```python
from build123d import *

# Parameters (mm, degrees)
EXTRUDE1_DEPTH  = 3
LPATTERN1_COUNT = 2
LPATTERN1_PITCH = 13.06


with BuildPart() as part:
    # Sketch1 → Extrude1 (new body)
    with BuildSketch(Plane(origin=(0, 0, 0), x_dir=(1, 0, 0), z_dir=(0, 1, 0))):
        Polygon((11.547005384, 0), (-5.773502692, 10), (-5.773502692, -10), align=None)
    extrude(amount=EXTRUDE1_DEPTH)

    # Sketch6 → #2-56 Tapped Hole1 (revolve, cut)
    with BuildSketch(Plane(origin=(-3.77, 3, -6.53), x_dir=(0, 0, 1), z_dir=(1, 0, 0))):
        Polygon((0, 0), (0, 7.17416509), (0.889, 6.64), (0.889, 0), align=None)
    f_2_56_tapped_hole1 = revolve(axis=Axis((-3.77, 9.35, -6.53), (0, -1, 0)), mode=Mode.SUBTRACT)

    # LPattern1: #2-56 Tapped Hole1 ×2
    with Locations(*[(0, 0, i * LPATTERN1_PITCH) for i in range(1, LPATTERN1_COUNT)]):
        add(f_2_56_tapped_hole1, mode=Mode.SUBTRACT)


solid = part.part
```
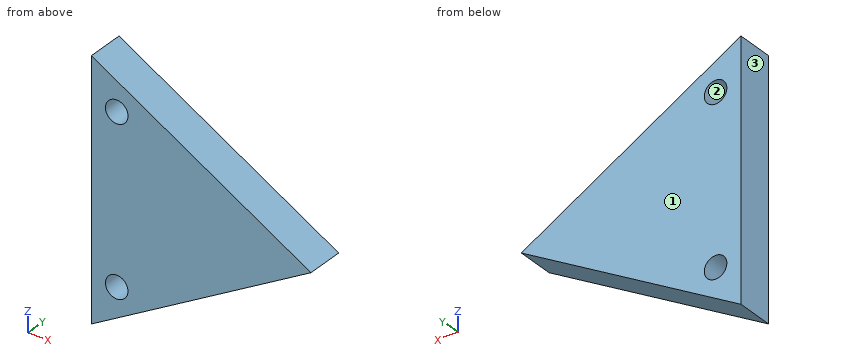
Model file for the job. Use its own axes, mm. Face numbers are marked on the shaded views. Coordinates: 2 decimals unless noted, no trailing zeros. Loops run counter-clockwise (first coordinate to the right, second up) from the corner with the lowest first, then second, coordinate; pieces in that order, holes last. Notation, with made-up numbers: (32, -23) - (64, -23) arc R30 cw to (64, 0) - close; hole circle Ø4 at (40, 70). An arc over 180 degrees is marked (long way). Write item = value, one per line. Start each with the question number.
Item 1: Saw through at C-C, the plane z = 6.5. List the corners of the cut face in (x, y), then the cut area to 3 significant figures.
Item 2: Pull direction X, two halves, no side cores. Call the marked faces 1, 2 and 3: +X half, -X half, draft (parallel to the pull), parting line (faces both ways), or undercut.
Item 3: Saw through at B-B, the plane x = -3.77. List the corners of the cut face in (y, z), then the cut area to 3 significant figures.
Item 4: Wall check: probe 1 along Z at (x, y) = (-3.77, 1.55); probe 2 along X at (y, z) = (1.6, 6.53); probe 3 along X at (y, z) = (1.6, 7.25). Give the ranges that are in metal, low to high. Write a range as [from, to].
Item 5: Saw through at D-D, the plane z = -2.75. List the corners of the cut face in (x, y), then the cut area to 3 significant figures.
Item 6: Drop flat-ended pins along their axis: pin 1 Ø1.6 at (x, z) = (-3.77, -6.53) entering from +Y; pin 2 Ø1.5 at (x, y) = (2.5, 1.5) entering from +Z; pin 3 Ø1 at (y, z) = (1, 4) entering from +X. Give the stop position or say it passes through.
Item 7: Saw through at A-A, the plane y = 1.2. List the corners of the cut face in (x, z).
Answers:
q1.outline = (-5.77, 0) - (-4.66, 0) - (-4.66, 3) - (-5.77, 3) - close; (-2.88, 0) - (0.29, 0) - (0.29, 3) - (-2.88, 3) - close
q1.area = 12.9 mm2
q2.face_1 = draft
q2.face_2 = undercut
q2.face_3 = -X half
q3.outline = (0, -8.84) - (3, -8.84) - (3, -7.42) - (0, -7.42) - close; (0, -5.64) - (3, -5.64) - (3, 5.64) - (0, 5.64) - close; (0, 7.42) - (3, 7.42) - (3, 8.84) - (0, 8.84) - close
q3.area = 42.4 mm2
q4.probe_1 = [-8.84, -7.42], [-5.64, 5.64], [7.42, 8.84]
q4.probe_2 = [-5.77, -4.66], [-2.88, 0.24]
q4.probe_3 = [-5.77, -4.29], [-3.25, -1.01]
q5.outline = (-5.77, 0) - (6.78, 0) - (6.78, 3) - (-5.77, 3) - close
q5.area = 37.7 mm2
q6.pin_1 = through
q6.pin_2 = 5.66
q6.pin_3 = 5.48
q7.outline = (-5.77, -10) - (11.55, 0) - (-5.77, 10) - close; hole circle Ø1.78 at (-3.77, -6.53); hole circle Ø1.78 at (-3.77, 6.53)
